```python
from build123d import *


with BuildPart() as part:
    # Sketch1 → Revolve1 (revolve)
    with BuildSketch(Plane(origin=(0, 0, 0), x_dir=(0, 0, -1), z_dir=(1, 0, 0)), mode=Mode.PRIVATE) as revolve1_sk:
        Polygon((0, 0), (0, 46.0375), (-12.7, 46.0375), (-12.7, 23.876), (-55.245, 23.876), (-55.245, 17.059549957), (-82.55, 17.059549957), (-82.55, 11.385820753), (-78.077653169, 4.7625), (-57.15, 4.7625), (-57.15, 0), align=None)
    revolve(revolve1_sk.sketch.rotate(Axis((0, 0, 57.15), (0, 0, -1)), 90), axis=Axis((0, 0, 57.15), (0, 0, -1)))


solid = part.part
```
Input: part model. Units: mm. Frame: model coordinates. A direction names the side the tool comes from. Coordinates: 2 decimals unless noted, no trailing zeros. Loops run counter-clockwise (first coordinate to the right, second up) from the corner with the lowest first, then second, coordinate; pieces in that order, holes last. Notation, with made-up numbers: (56.25, -12.5) - (106.25, -12.5) arc R23 ccw to (106.25, 19.5) - close; hole circle Ø10 at (33.25, -30.75). An arc over 180 degrees is marked (long way). Answer in a Markdown table with one row per item.
(1) Material intervals for L1, parallel to Y at x = 0, z = 69; L2, parallel to Z at x = 5, y = 30; L3, parallel to Z at x = -6, y = -21.5 (3 decimals), sorted ascending. Write a range as from..to.
Model answer:
| item | result |
|---|---|
| L1 | y = -17.06..-4.76, 4.76..17.06 |
| L2 | z = 0..12.7 |
| L3 | z = 0..55.245 |
(2) Cut plane D-D on x = 18.5. Output: boundary loops of the cut face in (y, z) (3 decimals), plus the area to 3 significant figures.
Model answer:
| item | result |
|---|---|
| outline | (-42.157, 0) - (42.157, 0) - (42.157, 12.7) - (15.093, 12.7) - (15.093, 55.245) - (-15.093, 55.245) - (-15.093, 12.7) - (-42.157, 12.7) - close |
| area | 2,360 mm² |
(3) Mould query, pull axis X, two halves, no side actions, for faces 1 (the face through (-1.03, 4.65, 67.47)), 2 (the face through (20, 20, 12.7)), 3 (the face through (-5.176, 23.308, 34.27)). Classes: pulls with the +X half, pulls with the -X half, needs draft (parallel to the pull), parting line crosses it, or undercut.
Model answer:
| item | result |
|---|---|
| face 1 | undercut |
| face 2 | needs draft |
| face 3 | parting line crosses it |
(4) Cut plane C-C on z = 50. Output: boundary loops of the cut face in (x, y), plus the area to 3 significant figures.
Model answer:
| item | result |
|---|---|
| outline | circle Ø47.75 at (0, 0) |
| area | 1,790 mm² |
(5) Set-up query: faces 4 (the face through (-16.3, -5.6, 55.245)), 5 (the face through (4, 11, 82.55)). Return all of +Z, -Z, +X, -X, +Y, -Y with unobstructed straight access to the full face (end or side cutting, diameter ignored); none if empty.
Model answer:
| item | result |
|---|---|
| face 4 | +Z |
| face 5 | +Z, +X, -X, +Y, -Y |
(6) Pin query (flat end, axial travel): P1, Ø10, axis at x = -12, z = 28.5, coming from the -Y side; P2, Ø4, axis at x = -7.5, y = 31.5, coming from the +Z side; P3, Ø1.5, axis at x = 18.5, z = 15.5, coming from the +Y side. Return the tip coordinate at first contact, or that it passes through.
Model answer:
| item | result |
|---|---|
| P1 | stops at y = -22.83 |
| P2 | stops at z = 12.7 |
| P3 | stops at y = 15.97 |
